Geometry check sheet. Reference: drawing and pictorial views, mm from the part's lowest x, y, z. A direction names the side the tool comes from. Round coordinates to 2 decimals unless told otherwise and drop trailing zeros. Write each loop counter-clockwise with the first axis right and the second up, starting at its lowest first coordinate (ties: lowest second). Pieces come first, ordered by that corner, then holes. Notation, with made-up numbers: M 43.5,-31.5 L 75.5,-31.5 A19 ccw 75.5,-21.5 Z; hole C 56,-14 d5. An arc over 180 degrees is marked long. One line per item, written item: value. Start each with the question number.
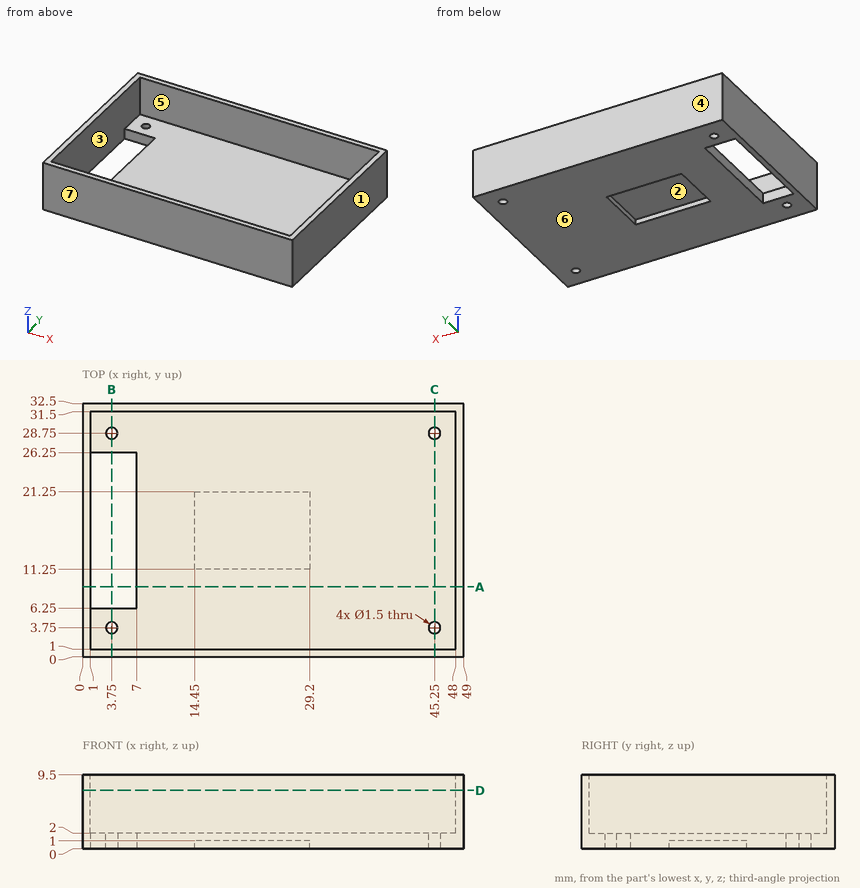
1) Cross-section at D-D (z = 7.5). Record the boundary of the cut face in (x, y), then the cut area to 3 significant figures.
2) Access from +Z, -Z, +X, -X, +Y, -Y to the whole of each face (thin tool, end or side, straight path). Record for the marked faces 1, 2 and 3.
3) Mould release check, pull along Y, two halves, no side actions. Record for the marked faces 4, 5, 6 and 7: pulls with the +Y half, pulls with the -Y half, needs draft (parallel to the pull), parting line crosses it, or undercut.
4) Gauge pin test, flat ends, axial feed: pin 1 Ø15 at (x, y) = (27.5, 21) entering from +Z; pin 2 Ø3 at (x, y) = (20.5, 15.5) entering from -Z. Record the tip position at first contact, or that the pin passes through.
5) Cross-section at C-C (x = 45.25). Record the boundary of the cut face in (y, z), then the cut area to 3 significant figures.
6) Cross-section at A-A (y = 9). Record the boundary of the cut face in (x, z).
7) Cross-section at B-B (x = 3.75). Record the boundary of the cut face in (y, z).
8) Thickness scan on line 1 (Y direction, x = 45.25, z = 0.9); line 2 (X direction, y = 25.5, z = 5.75); line 3 (Y direction, x = 39.5, z = 7). Record the ranges inside material, lowest first.
Results below:
1. outline: M 0,0 L 49,0 L 49,32.5 L 0,32.5 Z; hole M 1,1 L 48,1 L 48,31.5 L 1,31.5 Z
1. area: 159 mm²
2. face 1: +Z, -Z, +X, +Y, -Y
2. face 2: -Z
2. face 3: +Z
3. face 4: pulls with the +Y half
3. face 5: undercut
3. face 6: needs draft
3. face 7: pulls with the -Y half
4. pin 1: stops at z = 2
4. pin 2: stops at z = 1
5. outline: M 0,0 L 3,0 L 3,2 L 1,2 L 1,9.5 L 0,9.5 Z; M 4.5,0 L 28,0 L 28,2 L 4.5,2 Z; M 29.5,0 L 32.5,0 L 32.5,9.5 L 31.5,9.5 L 31.5,2 L 29.5,2 Z
5. area: 74.0 mm²
6. outline: M 0,0 L 1,0 L 1,9.5 L 0,9.5 Z; M 7,0 L 49,0 L 49,9.5 L 48,9.5 L 48,2 L 7,2 Z
7. outline: M 0,0 L 3,0 L 3,2 L 1,2 L 1,9.5 L 0,9.5 Z; M 4.5,0 L 6.25,0 L 6.25,2 L 4.5,2 Z; M 26.25,0 L 28,0 L 28,2 L 26.25,2 Z; M 29.5,0 L 32.5,0 L 32.5,9.5 L 31.5,9.5 L 31.5,2 L 29.5,2 Z
8. line 1: y = 0 to 3, 4.5 to 28, 29.5 to 32.5
8. line 2: x = 0 to 1, 48 to 49
8. line 3: y = 0 to 1, 31.5 to 32.5
